Geometry check sheet. Reference: the model listing, model coordinates, mm. Face numbers are marked on the shaded views. Give positions to 0.01 mm unless a question says otherwise; leave off trailing zeros. Write each loop counter-clockwise with the first axis right and the second up, starting at its lowest first coordinate (ties: lowest second). Pieces come first, ordered by that corner, then holes.
(1) Cross-section at A-A (z = 8). Count the separate pieces of the cut face and the enclosed holes in it, and give its area (3 significant figures).
(2) Cross-section at B-B (y = 18). Record the boundary of the cut face in (x, z), and give its area (3 significant figures).
(3) Depth check by flat-ended pin: P1, Ø4, axis at x = 51.5, z = 8, coming from the +Y side; P2, Ø2, axis at y = 49.5, z = 3.5, coming from the -X side; P3, Ø5, axis at x = 46.5, z = 5.5, coming from the -Y side. Enter the tip coordinate at first touch or a pass-through.
(4) Mould release check, pull along X, two halves, no side actions. Record for the marked faces 1, 2 and 3: +X half, -X half, draft (parallel to the pull), parting line (faces both ways), or undercut.
(5) Thickness scan on line 1 along Y through (x, z) = (0, 9.75); line 2 along Y through (x, z) = (0, 2.2); line 3 along Y through (x, z) = (27.5, 5.25). Record the ranges inside material, lowest first.
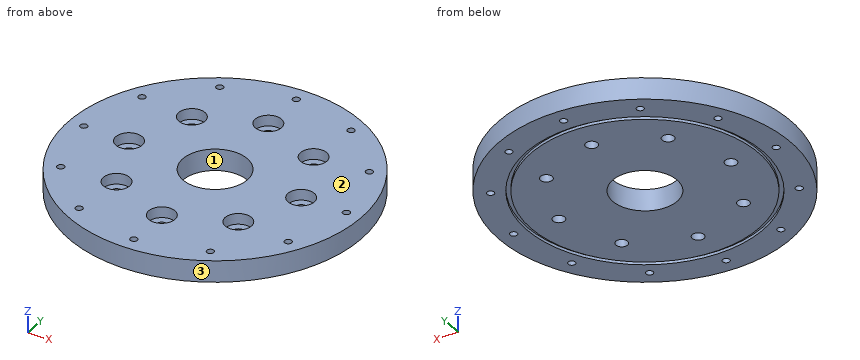
```python
from build123d import *

# Parameters (mm, degrees)
SKETCH1_R                               = 75
BOSS_EXTRUDE1_DEPTH                     = 10
SKETCH3_R                               = 15
CUT_EXTRUDE2_DEPTH                      = 10
SKETCH8_R                               = 55
SKETCH8_R_2                             = 53
CUT_EXTRUDE7_DEPTH                      = 1.3208
CBORE_FOR_M5_HEX_HEAD_BOLT1_D           = 5.5
CBORE_FOR_M5_HEX_HEAD_BOLT1_CBORE_D     = 12.238
CBORE_FOR_M5_HEX_HEAD_BOLT1_CBORE_DEPTH = 3.5
SKETCH11_R                              = 75
SKETCH11_R_2                            = 68
CUT_EXTRUDE8_DEPTH                      = 10
SKETCH12_R                              = 6.119
CUT_EXTRUDE9_DEPTH                      = 5
CIRPATTERN2_COUNT                       = 8
M4_TAPPED_HOLE1_D                       = 3.3
CIRPATTERN3_COUNT                       = 12


with BuildPart() as part:
    # Sketch1 → Boss-Extrude1 (new body)
    with BuildSketch(Plane.XY):
        Circle(SKETCH1_R)
    extrude(amount=BOSS_EXTRUDE1_DEPTH)

    # Sketch3 → Cut-Extrude2 (cut)
    with BuildSketch(Plane.XY.offset(10)):
        Circle(SKETCH3_R)
    extrude(amount=-CUT_EXTRUDE2_DEPTH, mode=Mode.SUBTRACT)

    # Sketch8 → Cut-Extrude7 (cut)
    with BuildSketch(Plane.XY):
        Circle(SKETCH8_R)
        Circle(SKETCH8_R_2, mode=Mode.SUBTRACT)
    extrude(amount=CUT_EXTRUDE7_DEPTH, mode=Mode.SUBTRACT)

    # CBORE for M5 Hex Head Bolt1 (through all)
    with Locations(Plane.XY.offset(10)):
        with Locations((28.284271247, 28.284271247)):
            cbore_for_m5_hex_head_bolt1 = CounterBoreHole(CBORE_FOR_M5_HEX_HEAD_BOLT1_D / 2, CBORE_FOR_M5_HEX_HEAD_BOLT1_CBORE_D / 2, CBORE_FOR_M5_HEX_HEAD_BOLT1_CBORE_DEPTH)

    # Sketch11 → Cut-Extrude8 (cut)
    with BuildSketch(Plane.XY.offset(10)):
        Circle(SKETCH11_R)
        Circle(SKETCH11_R_2, mode=Mode.SUBTRACT)
    extrude(amount=-CUT_EXTRUDE8_DEPTH, mode=Mode.SUBTRACT)

    # Sketch12 → Cut-Extrude9 (cut)
    with BuildSketch(Plane.XY.offset(10)):
        with Locations((28.284271247, 28.284271247)):
            Circle(SKETCH12_R)
    cut_extrude9 = extrude(amount=-CUT_EXTRUDE9_DEPTH, mode=Mode.SUBTRACT)

    # CirPattern2: CBORE for M5 Hex Head Bolt1, Cut-Extrude9 ×8 about axis
    cirpattern2_axis = Axis((0, 0, 0), (0, 0, 1))
    for i in range(1, CIRPATTERN2_COUNT):
        add(cbore_for_m5_hex_head_bolt1.rotate(cirpattern2_axis, i * 360 / CIRPATTERN2_COUNT), mode=Mode.SUBTRACT)
        add(cut_extrude9.rotate(cirpattern2_axis, i * 360 / CIRPATTERN2_COUNT), mode=Mode.SUBTRACT)

    # M4 Tapped Hole1 (through all)
    with Locations(Plane.XY.offset(10)):
        with Locations((0, 61)):
            m4_tapped_hole1 = Hole(M4_TAPPED_HOLE1_D / 2)

    # CirPattern3: M4 Tapped Hole1 ×12 about axis
    cirpattern3_axis = Axis((0, 0, 0), (0, 0, 1))
    for i in range(1, CIRPATTERN3_COUNT):
        add(m4_tapped_hole1.rotate(cirpattern3_axis, i * 360 / CIRPATTERN3_COUNT), mode=Mode.SUBTRACT)


solid = part.part
```
Reply:
1. separate pieces: 1
1. enclosed holes: 21
1. area: 12,800 mm2
2. outline: (-65.57, 0) - (-51.97, 0) - (-51.97, 1.32) - (-49.85, 1.32) - (-49.85, 0) - (49.85, 0) - (49.85, 1.32) - (51.97, 1.32) - (51.97, 0) - (65.57, 0) - (65.57, 10) - (-65.57, 10) - close
2. area: 1,310 mm2
3. P1: stops at y = 46.62
3. P2: stops at x = -47.66
3. P3: stops at y = -51.85
4. face 1: undercut
4. face 2: draft
4. face 3: parting line
5. line 1: y = -68 to -62.65, -59.35 to -46.12, -33.88 to -15, 15 to 33.88, 46.12 to 59.35, 62.65 to 68
5. line 2: y = -68 to -62.65, -59.35 to -42.75, -37.25 to -15, 15 to 37.25, 42.75 to 59.35, 62.65 to 68
5. line 3: y = -62.19 to -34.35, -22.22 to 22.22, 34.35 to 62.19
